```python
from build123d import *

# Parameters (mm, degrees)
ESQUISSE1_R        = 4
BOSS_EXTRU_1_DEPTH = 1050


with BuildPart() as part:
    # Esquisse1 → Boss.-Extru.1 (new body)
    with BuildSketch(Plane(origin=(0, 0, -1000), x_dir=(-1, 0, 0), z_dir=(0, 0, -1))):
        with BuildLine():
            Line((16.5, 26.5), (22.5, 26.5))
            Line((22.5, 26.5), (22.5, 42))
            ThreePointArc((22.5, 42), (21.621320344, 44.121320344), (19.5, 45))
            Line((19.5, 45), (4, 45))
            Line((4, 45), (4, 39))
            Line((4, 39), (-4, 39))
            Line((-4, 39), (-4, 45))
            Line((-4, 45), (-19.5, 45))
            ThreePointArc((-19.5, 45), (-21.621320344, 44.121320344), (-22.5, 42))
            Line((-22.5, 42), (-22.5, 26.5))
            Line((-22.5, 26.5), (-16.5, 26.5))
            Line((-16.5, 26.5), (-16.5, 18.5))
            Line((-16.5, 18.5), (-22.5, 18.5))
            Line((-22.5, 18.5), (-22.5, -18.5))
            Line((-22.5, -18.5), (-16.5, -18.5))
            Line((-16.5, -18.5), (-16.5, -26.5))
            Line((-16.5, -26.5), (-22.5, -26.5))
            Line((-22.5, -26.5), (-22.5, -42))
            ThreePointArc((-22.5, -42), (-21.621320344, -44.121320344), (-19.5, -45))
            Line((-19.5, -45), (-4, -45))
            Line((-4, -45), (-4, -39))
            Line((-4, -39), (4, -39))
            Line((4, -39), (4, -45))
            Line((4, -45), (19.5, -45))
            ThreePointArc((19.5, -45), (21.621320344, -44.121320344), (22.5, -42))
            Line((22.5, -42), (22.5, -26.5))
            Line((22.5, -26.5), (16.5, -26.5))
            Line((16.5, -26.5), (16.5, -18.5))
            Line((16.5, -18.5), (22.5, -18.5))
            Line((22.5, -18.5), (22.5, 18.5))
            Line((22.5, 18.5), (16.5, 18.5))
            Line((16.5, 18.5), (16.5, 26.5))
        make_face()
        with Locations((0, 22.5)):
            Circle(ESQUISSE1_R, mode=Mode.SUBTRACT)
        with Locations((0, -22.5)):
            Circle(ESQUISSE1_R, mode=Mode.SUBTRACT)
    extrude(amount=-BOSS_EXTRU_1_DEPTH)


solid = part.part
```
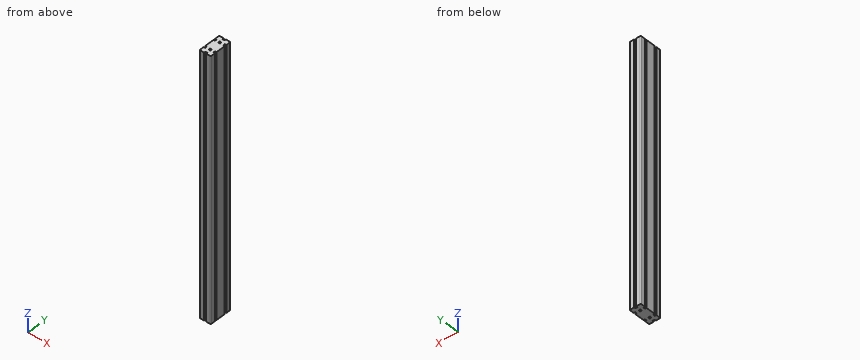
The model under review builds one solid part; all positions refer to its coordinate system, in mm. Round coordinates to 2 decimals unless told otherwise and drop trailing zeros.
(1) Wall thickness on L1, parallel to Y at x = -18, z = -491; L2, parallel to Y at x = 0, z = -504; L3, parallel to X at y = 22, z = -586: over which ranges is each line inside the solid? List them lowest first.
(2) Insertion check: pin 1 (1.8 mm diameter, centred on x = -21, z = -589.5, fed in from +Y); pin 2 (2.5 mm diameter, centred on x = -1, z = -311, fed in from -Y); pin 3 (1 mm diameter, centred on x = 3, z = -748, fed in from +Y). Each pin has a flat end and moves straight along its axis. Give the tip position at first contact, or say it passes through.
(3) We need section A-A on z = -279.5. Give the number of separate pieces and of enclosed holes in the cut face, and give its area (3 significant figures).
Findings below:
1. L1: y = -45 to -26.5, -18.5 to 18.5, 26.5 to 45
1. L2: y = -39 to -26.5, -18.5 to 18.5, 26.5 to 39
1. L3: x = -16.5 to -3.97, 3.97 to 16.5
2. pin 1: stops at y = 44.94
2. pin 2: stops at y = -39
2. pin 3: stops at y = 39
3. separate pieces: 1
3. enclosed holes: 2
3. area: 3,650 mm2
